```python
from build123d import *

# Parameters (mm, degrees)
SKETCH1_W                      = 35.5
SKETCH1_H                      = 12.5
BOSS_EXTRUDE1_DEPTH            = 10
SKETCH2_W                      = 25.5
SKETCH2_H                      = 7.5
CUT_EXTRUDE1_DEPTH             = 7.5
SKETCH4_R                      = 1
CUT_EXTRUDE2_DEPTH             = 4
SKETCH6_W                      = 9
SKETCH6_H                      = 2.5
CUT_EXTRUDE3_DEPTH             = 4
CUT_EXTRUDE4_REACH             = 12
SKETCH7_R                      = 1.6
CUT_EXTRUDE4_DIRECTION_2_DEPTH = 1


with BuildPart() as part:
    # Sketch1 → Boss-Extrude1 (new body)
    with BuildSketch(Plane(origin=(0, 0, 0), x_dir=(1, 0, 0), z_dir=(0, 1, 0))):
        Rectangle(SKETCH1_W, SKETCH1_H)
    extrude(amount=BOSS_EXTRUDE1_DEPTH)

    # Sketch2 → Cut-Extrude1 (cut)
    with BuildSketch(Plane.XZ):
        with Locations((0, -2.5)):
            Rectangle(SKETCH2_W, SKETCH2_H)
    extrude(amount=-CUT_EXTRUDE1_DEPTH, mode=Mode.SUBTRACT)

    # Sketch4 → Cut-Extrude2 (cut)
    with BuildSketch(Plane(origin=(0, 0, -6.25), x_dir=(-1, 0, 0), z_dir=(0, 0, -1))):
        with Locations((-14.75, 3)):
            Circle(SKETCH4_R)
        with Locations((14.75, 3)):
            Circle(SKETCH4_R)
    extrude(amount=-CUT_EXTRUDE2_DEPTH, mode=Mode.SUBTRACT)

    # Sketch6 → Cut-Extrude3 (cut)
    with BuildSketch(Plane(origin=(0, 0, -6.25), x_dir=(-1, 0, 0), z_dir=(0, 0, -1))):
        with Locations((8.25, 8.75)):
            Rectangle(SKETCH6_W, SKETCH6_H)
    extrude(amount=-CUT_EXTRUDE3_DEPTH, mode=Mode.SUBTRACT)

    # Sketch7 → Cut-Extrude4 (cut, up to next)
    with BuildSketch(Plane(origin=(0, 10, 0), x_dir=(1, 0, 0), z_dir=(0, 1, 0)), mode=Mode.PRIVATE) as cut_extrude4_sk1:
        with Locations((-0.75, 4.25)):
            Circle(SKETCH7_R)
    cut_extrude4_tool1 = extrude(cut_extrude4_sk1.sketch, amount=-CUT_EXTRUDE4_REACH, mode=Mode.PRIVATE) & part.part
    add(cut_extrude4_tool1.solids().sort_by_distance((-0.75, 10, -4.25))[0], mode=Mode.SUBTRACT)

    # Sketch7 → Cut-Extrude4 direction 2 (cut)
    with BuildSketch(Plane(origin=(0, 10, 0), x_dir=(1, 0, 0), z_dir=(0, 1, 0))):
        with Locations((-0.75, 4.25)):
            Circle(SKETCH7_R)
    extrude(amount=CUT_EXTRUDE4_DIRECTION_2_DEPTH, mode=Mode.SUBTRACT)


solid = part.part
```
Design review of the part built by this model. Coordinates are the model's own, in mm. A direction names the side the tool comes from. Give positions to 0.01 mm unless a question says otherwise; leave off trailing zeros. Write each loop counter-clockwise with the first axis right and the second up, starting at its lowest first coordinate (ties: lowest second). Pieces come first, ordered by that corner, then holes. Notation, with made-up numbers: (-15.5, 32) - (32.5, 32) arc R33 cw to (32.5, 70) - close; hole circle Ø1 at (61, -25.75). An arc over 180 degrees is marked (long way). Return JSON: item names as keys, results as strings. Group by question number.
(1) We need section D-D, the plane x = -14.75. Give the boundary of the cut face in (y, z), then the cut area to 3 significant figures.
(2) We need section B-B, the plane x = -0.75. Give the boundary of the cut face in (y, z), then the cut area to 4 significant figures.
(3) Machinability: for faces 1 (the flat face through (-12.75, 5, -3)), 2 (the flat face through (-8, 9, -2.25)), 3 (the flat face through (15, 3, -2.25)), which of the approach directions +Z, -Z, +X, -X, +Y, -Y give a long, thin tool a straight path to every point of the face, cutting with its end or side? Answer none if there is none.
(4) We need section A-A, the plane z = -4.25. Give the boundary of the cut face in (x, y), then the cut area to 3 significant figures.
(5) To check wall thickness, follow probe 1 along Z at (x, y) = (-0.75, 8.45); probe 2 along X at (y, z) = (3.25, -0.75); probe 3 along X at (y, z) = (8.05, -4.25). State the ranges of each line that lie inside material, in increasing order.
(6) We need section C-C, the plane y = 8.75. Give the boundary of the cut face in (x, z).
(7) Mouldability with a two-part tool opening along X and no side actions: class faces 4 (the flat face through (0, 4, 1.25)), 5 (the flat face through (0, 0, 3)), 6 (the flat face through (17.75, 5, 0)), 7 (the flat face through (-17.75, 5, 0)) as +X half, -X half, draft (parallel to the pull), parting line (faces both ways), or undercut.
(8) Insertion check: pin 1 (4 mm diameter, centred on x = -2, z = -3.5, fed in from -Y); pin 2 (2 mm diameter, centred on x = -15, y = 3, fed in from -Z); pin 3 (1.8 mm diameter, centred on x = -14.75, y = 3, fed in from -Z). Each pin has a flat end and moves straight along its axis. Give the tip position at first contact, or say it passes through.
Reported:
{
 "1": {"outline": "(0, -6.25) - (2, -6.25) - (2, -2.25) - (4, -2.25) - (4, -6.25) - (10, -6.25) - (10, 6.25) - (0, 6.25) - close", "area": "117 mm2"},
 "2": {"outline": "(0, 1.25) - (7.5, 1.25) - (7.5, -2.65) - (10, -2.65) - (10, 6.25) - (0, 6.25) - close; (7.5, -6.25) - (10, -6.25) - (10, -5.85) - (7.5, -5.85) - close", "area": "60.75 mm2"},
 "3": {"face 1": "-Z, -Y", "face 2": "-Z, +Y, -Y", "face 3": "-Z"},
 "4": {"outline": "(-17.75, 0) - (-12.75, 0) - (-12.75, 10) - (-17.75, 10) - close; (-3.75, 7.5) - (-2.35, 7.5) - (-2.35, 10) - (-3.75, 10) - close; (0.85, 7.5) - (12.75, 7.5) - (12.75, 0) - (17.75, 0) - (17.75, 10) - (0.85, 10) - close; hole circle Ø2 at (-14.75, 3); hole circle Ø2 at (14.75, 3)", "area": "127 mm2"},
 "5": {"probe 1": "z = -6.25 to -5.85, -2.65 to 6.25", "probe 2": "x = -17.75 to -12.75, 12.75 to 17.75", "probe 3": "x = -17.75 to -12.75, -3.75 to -2.35, 0.85 to 17.75"},
 "6": {"outline": "(-17.75, -6.25) - (-12.75, -6.25) - (-12.75, -2.25) - (-3.75, -2.25) - (-3.75, -6.25) - (17.75, -6.25) - (17.75, 6.25) - (-17.75, 6.25) - close; hole circle Ø3.2 at (-0.75, -4.25)"},
 "7": {"face 4": "undercut", "face 5": "draft", "face 6": "+X half", "face 7": "-X half"},
 "8": {"pin 1": "stops at y = 7.5", "pin 2": "stops at z = -6.25", "pin 3": "stops at z = -2.25"}
}
